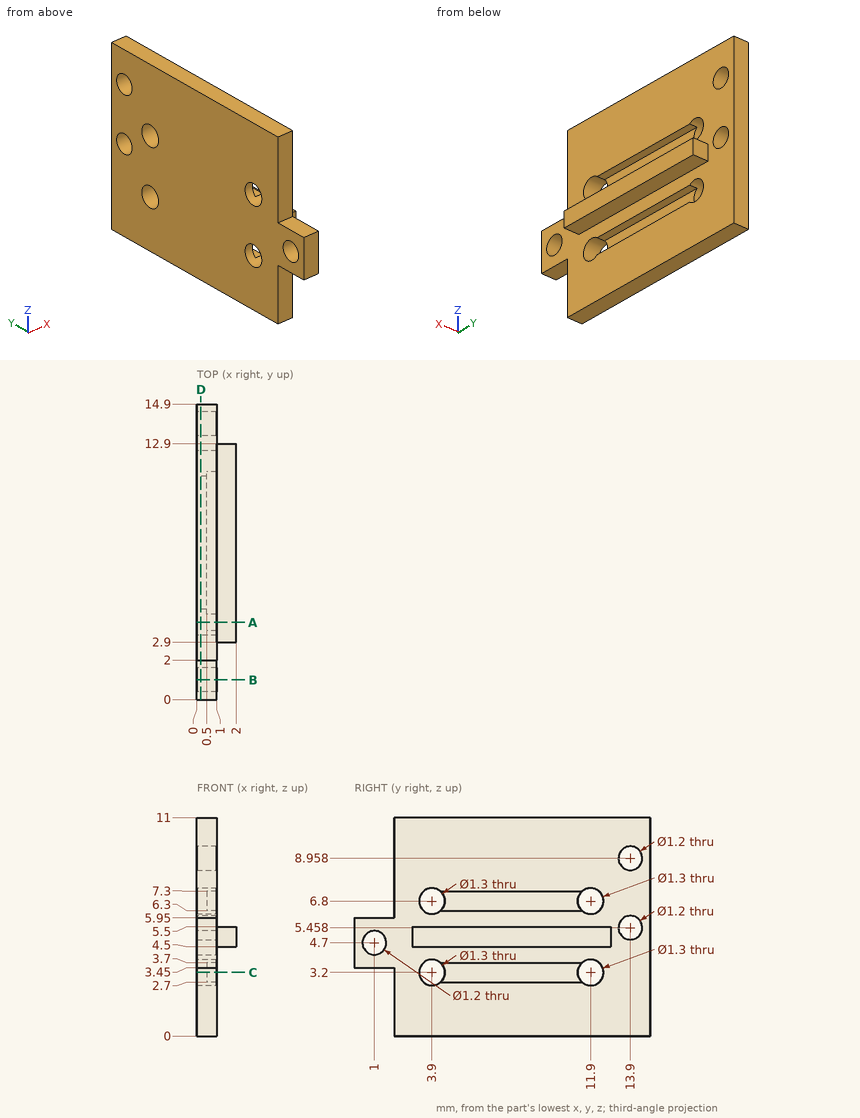
The drawing under review shows one solid part. Ordinate dimensions are in mm from its lowest x, y, z. Give positions to 0.01 mm unless a question says otherwise; leave off trailing zeros. Loops run counter-clockwise (first coordinate to the right, second up) from the corner with the lowest first, then second, coordinate; pieces in that order, holes last. Notation, with made-up numbers: M 22,22.25 L 32,22.25 A19 ccw 32,40.25 Z; hole C -26,22.25 d5. An arc over 180 degrees is marked long. One line per item, written item: value. Start each with the question number.
Q1. For L1, parallel to Z at x = 0.3, y = 11.9; L2, parallel to Y at x = 0.35, z = 3.2; L3, parallel to Y at x = 0.8, z = 3.2, list the stretches that pass through material, from the lowest coordinate up.
Q2. Add section A-A (y = 3.9). Give the boundary of the cut face in (x, z).
Q3. Add section C-C (z = 3.2). Give the boundary of the cut face in (x, y).
Q4. Add section D-D (x = 0.2). Give the boundary of the cut face in (y, z), and give its area (3 significant figures).
Q5. Add section B-B (y = 1). Give the boundary of the cut face in (x, z).
Q6. Clearance check with flat-ended pins moving along their axes: pin 1 Ø1.2 at (y, z) = (3.9, 6.8) entering from +X; pin 2 Ø1.1 at (y, z) = (6.5, 3.5) entering from +X; pin 3 Ø1.1 at (x, z) = (0.5, 8.5) entering from -Y. State where each tip first meets the part, or that it passes through.
Reply:
1. L1: 0 to 2.55, 3.85 to 6.15, 7.45 to 11
1. L2: 2 to 3.25, 4.55 to 11.25, 12.55 to 14.9
1. L3: 2 to 3.25, 12.55 to 14.9
2. outline: M 0,0 L 1,0 L 1,2.55 L 0,2.55 Z; M 0,3.85 L 1,3.85 L 1,4.5 L 2,4.5 L 2,5.5 L 1,5.5 L 1,6.15 L 0,6.15 Z; M 0,7.45 L 1,7.45 L 1,11 L 0,11 Z
3. outline: M 0,2 L 1,2 L 1,3.25 L 0,3.25 Z; M 0,4.55 L 0.5,4.55 L 0.5,11.25 L 0,11.25 Z; M 0,12.55 L 1,12.55 L 1,14.9 L 0,14.9 Z
4. outline: M 0,3.45 L 2,3.45 L 2,0 L 14.9,0 L 14.9,11 L 2,11 L 2,5.95 L 0,5.95 Z; hole C 1,4.7 d1.2; hole C 3.9,3.2 d1.3; hole C 3.9,6.8 d1.3; hole C 11.9,3.2 d1.3; hole C 11.9,6.8 d1.3; hole C 13.9,5.46 d1.2; hole C 13.9,8.96 d1.2
4. area: 138 mm²
5. outline: M 0,3.45 L 1,3.45 L 1,4.1 L 0,4.1 Z; M 0,5.3 L 1,5.3 L 1,5.95 L 0,5.95 Z
6. pin 1: through
6. pin 2: x = 1
6. pin 3: y = 2
